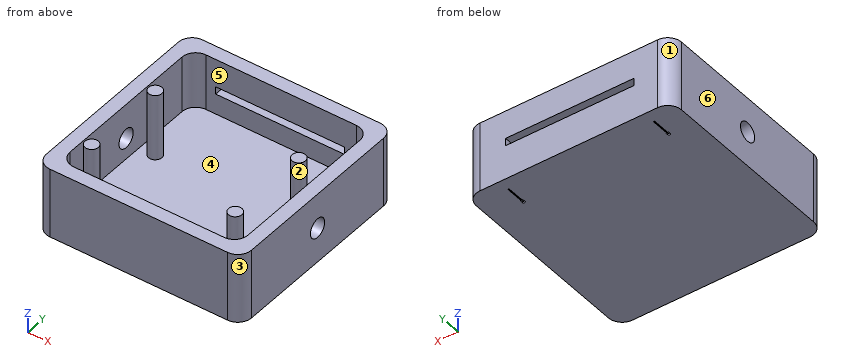
```python
from build123d import *

# Parameters (mm, degrees)
SKETCH1_W           = 30
SKETCH1_H           = 30
BOSS_EXTRUDE1_DEPTH = 2
SKETCH4_R           = 0.9775
BOSS_EXTRUDE3_DEPTH = 9.7
SKETCH5_W           = 30
SKETCH5_H           = 30
SKETCH5_W_2         = 26
SKETCH5_H_2         = 26
BOSS_EXTRUDE4_DEPTH = 8.25
SKETCH6_W           = 18.8
SKETCH6_H           = 1.1
CUT_EXTRUDE1_DEPTH  = 10
FILLET1_R           = 2
CUT_EXTRUDE4_DEPTH  = 0.25
BOSS_EXTRUDE6_DEPTH = 0.05
CUT_EXTRUDE5_DEPTH  = 0.25
BOSS_EXTRUDE7_DEPTH = 0.05
SKETCH23_R          = 1.4
CUT_EXTRUDE6_DEPTH  = 3
CUT_EXTRUDE7_START  = -3
SKETCH24_R          = 1.4
CUT_EXTRUDE7_DEPTH  = 3


with BuildPart() as part:
    # Sketch1 → Boss-Extrude1 (new body)
    with BuildSketch(Plane.XY):
        with Locations((-5.423452769, 0.244299674)):
            Rectangle(SKETCH1_W, SKETCH1_H)
    extrude(amount=BOSS_EXTRUDE1_DEPTH)

    # Sketch4 → Boss-Extrude3 (add)
    with BuildSketch(Plane.XY.offset(2)):
        with Locations((-16.173452769, 2.943299674)):
            Circle(SKETCH4_R)
        with Locations((-16.173452769, -9.555700326)):
            Circle(SKETCH4_R)
        with Locations((4.826547231, 2.943299674)):
            Circle(SKETCH4_R)
        with Locations((4.826547231, -9.555700326)):
            Circle(SKETCH4_R)
    extrude(amount=BOSS_EXTRUDE3_DEPTH)

    # Sketch5 → Boss-Extrude4 (add)
    with BuildSketch(Plane.XY.offset(2)):
        with Locations((-5.423452769, 0.244299674)):
            Rectangle(SKETCH5_W, SKETCH5_H)
        with Locations((-5.423452769, 0.244299674)):
            Rectangle(SKETCH5_W_2, SKETCH5_H_2, mode=Mode.SUBTRACT)
    extrude(amount=BOSS_EXTRUDE4_DEPTH)

    # Sketch6 → Cut-Extrude1 (cut)
    with BuildSketch(Plane(origin=(0, 15.244299674, 0), x_dir=(1, 0, 0), z_dir=(0, 1, 0))):
        with Locations((-5.582175382, -5.564963199)):
            Rectangle(SKETCH6_W, SKETCH6_H)
    extrude(amount=-CUT_EXTRUDE1_DEPTH, mode=Mode.SUBTRACT)

    # Fillet1
    fillet1_edges = [part.edges().sort_by_distance(p)[0] for p in [
        (7.576547231, 13.244299674, 6.125),
        (7.576547231, -12.755700326, 6.125),
        (-18.423452769, -12.755700326, 6.125),
        (-18.423452769, 13.244299674, 6.125),
        (-20.423452769, 15.244299674, 5.125),
        (9.576547231, 15.244299674, 5.125),
        (9.576547231, -14.755700326, 5.125),
        (-20.423452769, -14.755700326, 5.125),
    ]]
    fillet(fillet1_edges, radius=FILLET1_R)

    # Sketch15 → Cut-Extrude4 (cut)
    with BuildSketch(Plane(origin=(0, 0, 0), x_dir=(-1, 0, 0), z_dir=(0, 0, -1))):
        with BuildLine():
            Line((-4.48872314, 13.480732705), (-4.48872314, 10.524770746))
            ThreePointArc((-4.48872314, 10.524770746), (-4.67872314, 10.334770746), (-4.86872314, 10.524770746))
            Line((-4.86872314, 10.524770746), (-4.86872314, 13.480732705))
            ThreePointArc((-4.86872314, 13.480732705), (-4.67872314, 13.670732705), (-4.48872314, 13.480732705))
        make_face()
    extrude(amount=-CUT_EXTRUDE4_DEPTH, mode=Mode.SUBTRACT)

    # Sketch16 → Boss-Extrude6 (add)
    with BuildSketch(Plane(origin=(0, 0, 0), x_dir=(-1, 0, 0), z_dir=(0, 0, -1))):
        with BuildLine():
            Line((-4.86872314, 10.923343064), (-4.772315146, 10.923343064))
            Line((-4.772315146, 10.923343064), (-4.772315146, 13.480732705))
            ThreePointArc((-4.772315146, 13.480732705), (-4.68554888, 13.567498971), (-4.598782614, 13.480732705))
            Line((-4.598782614, 13.480732705), (-4.598782614, 10.923343064))
            Line((-4.598782614, 10.923343064), (-4.48872314, 10.923343064))
            Line((-4.48872314, 10.923343064), (-4.48872314, 13.480732705))
            ThreePointArc((-4.48872314, 13.480732705), (-4.67872314, 13.670732705), (-4.86872314, 13.480732705))
            Line((-4.86872314, 13.480732705), (-4.86872314, 10.923343064))
        make_face()
    extrude(amount=-BOSS_EXTRUDE6_DEPTH)

    # Sketch20 → Cut-Extrude5 (cut)
    with BuildSketch(Plane(origin=(0, 0, 0), x_dir=(-1, 0, 0), z_dir=(0, 0, -1))):
        with BuildLine():
            Line((16.739959819, 13.377498971), (16.739959819, 10.515388846))
            ThreePointArc((16.739959819, 10.515388846), (16.549959819, 10.325388846), (16.359959819, 10.515388846))
            Line((16.359959819, 10.515388846), (16.359959819, 13.377498971))
            ThreePointArc((16.359959819, 13.377498971), (16.549959819, 13.567498971), (16.739959819, 13.377498971))
        make_face()
    extrude(amount=-CUT_EXTRUDE5_DEPTH, mode=Mode.SUBTRACT)

    # Sketch19 → Boss-Extrude7 (add)
    with BuildSketch(Plane(origin=(0, 0, 0), x_dir=(-1, 0, 0), z_dir=(0, 0, -1))):
        with BuildLine():
            Line((16.359959819, 10.82010933), (16.456367814, 10.82010933))
            Line((16.456367814, 10.82010933), (16.456367814, 13.377498971))
            ThreePointArc((16.456367814, 13.377498971), (16.543134079, 13.464265237), (16.629900345, 13.377498971))
            Line((16.629900345, 13.377498971), (16.629900345, 10.82010933))
            Line((16.629900345, 10.82010933), (16.739959819, 10.82010933))
            Line((16.739959819, 10.82010933), (16.739959819, 13.377498971))
            ThreePointArc((16.739959819, 13.377498971), (16.549959819, 13.567498971), (16.359959819, 13.377498971))
            Line((16.359959819, 13.377498971), (16.359959819, 10.82010933))
        make_face()
    extrude(amount=-BOSS_EXTRUDE7_DEPTH)

    # Sketch23 → Cut-Extrude6 (cut)
    with BuildSketch(Plane.ZY.offset(20.423452769)):
        with Locations((5.125, 0.244299674)):
            Circle(SKETCH23_R)
    extrude(amount=-CUT_EXTRUDE6_DEPTH, mode=Mode.SUBTRACT)

    # Sketch24 → Cut-Extrude7 (cut)
    with BuildSketch(Plane(origin=(9.576547231, 0, 0), x_dir=(0, 0, -1), z_dir=(1, 0, 0)).offset(CUT_EXTRUDE7_START)):
        with Locations(Location((-5.125, 0.244299674, 0), (0, 0, 180))):
            Circle(SKETCH24_R)
    extrude(amount=CUT_EXTRUDE7_DEPTH, mode=Mode.SUBTRACT)


solid = part.part
```
Input: part model. Units: mm. Frame: model coordinates. Face numbers are marked on the shaded views. A direction names the side the tool comes from. Coordinates: 2 decimals unless noted, no trailing zeros. Loops run counter-clockwise (first coordinate to the right, second up) from the corner with the lowest first, then second, coordinate; pieces in that order, holes last. Notation, with made-up numbers: (54.25, 5.5) - (108.25, 5.5) arc R17 ccw to (108.25, 23.5) - close; hole circle Ø9 at (3, -6). An arc over 180 degrees is marked (long way). Answer in a Markdown table with one row per item.
(1) Cut plane A-A on x = -11.75. Output: boundary loops of the cut face in (y, z).
Model answer:
| item | result |
|---|---|
| outline | (-14.76, 0) - (15.24, 0) - (15.24, 5.01) - (13.24, 5.01) - (13.24, 2) - (-12.76, 2) - (-12.76, 10.25) - (-14.76, 10.25) - close; (13.24, 6.11) - (15.24, 6.11) - (15.24, 10.25) - (13.24, 10.25) - close |
(2) Mould query, pull axis X, two halves, no side actions, for the marked faces 1, 2, 3 and 4. Classes: pulls with the +X half, pulls with the -X half, needs draft (parallel to the pull), parting line crosses it, or undercut.
Model answer:
| item | result |
|---|---|
| face 1 | pulls with the -X half |
| face 2 | undercut |
| face 3 | pulls with the +X half |
| face 4 | undercut |
(3) Cut plane C-C on y = -4. Output: boundary loops of the cut face in (x, z).
Model answer:
| item | result |
|---|---|
| outline | (-20.42, 0) - (9.58, 0) - (9.58, 10.25) - (7.58, 10.25) - (7.58, 2) - (-18.42, 2) - (-18.42, 10.25) - (-20.42, 10.25) - close |
(4) Pin query (flat end, axial travel): P1, Ø8, axis at x = -6, y = -3.5, coming from the +Z side; P2, Ø2, axis at y = 0.24, z = 5.12, coming from the -X side; P3, Ø6, axis at x = -4, y = -11, coming from the +Z side; P4, Ø0.5, axis at y = 14.5, z = 5.5, coming from the +X side. Return the tip coordinate at first contact, or that it passes through.
Model answer:
| item | result |
|---|---|
| P1 | stops at z = 2 |
| P2 | passes through |
| P3 | stops at z = 10.25 |
| P4 | stops at x = 9.31 |
(5) Cut plane D-D on z = 4.25. Output: boundary loops of the cut face in (x, y) (1 decimal).
Model answer:
| item | result |
|---|---|
| outline | (-20.4, -12.8) arc R2 ccw to (-18.4, -14.8) - (7.6, -14.8) arc R2 ccw to (9.6, -12.8) - (9.6, -0.8) - (7.6, -0.8) - (7.6, -10.8) arc R2 cw to (5.6, -12.8) - (-16.4, -12.8) arc R2 cw to (-18.4, -10.8) - (-18.4, -0.8) - (-20.4, -0.8) - close; (-20.4, 1.3) - (-18.4, 1.3) - (-18.4, 11.2) arc R2 cw to (-16.4, 13.2) - (5.6, 13.2) arc R2 cw to (7.6, 11.2) - (7.6, 1.3) - (9.6, 1.3) - (9.6, 13.2) arc R2 ccw to (7.6, 15.2) - (-18.4, 15.2) arc R2 ccw to (-20.4, 13.2) - close; circle Ø2 at (-16.2, -9.6); circle Ø2 at (-16.2, 2.9); circle Ø2 at (4.8, -9.6); circle Ø2 at (4.8, 2.9) |
(6) Material intervals for L1, parallel to X at y = -2.5, z = 5.75; L2, parallel to Y at x = 0, z = 10; L3, parallel to Y at x = -15.5, z = 8.5, sorted ascending. Write a range as from..to.
Model answer:
| item | result |
|---|---|
| L1 | x = -20.42..-18.42, 7.58..9.58 |
| L2 | y = -14.76..-12.76, 13.24..15.24 |
| L3 | y = -14.76..-12.76, -10.26..-8.85, 2.23..3.65, 13.24..15.24 |
(7) Cut plane B-B on z = 9. Output: boundary loops of the cut face in (x, y) (1 decimal).
Model answer:
| item | result |
|---|---|
| outline | (-20.4, -12.8) arc R2 ccw to (-18.4, -14.8) - (7.6, -14.8) arc R2 ccw to (9.6, -12.8) - (9.6, 13.2) arc R2 ccw to (7.6, 15.2) - (-18.4, 15.2) arc R2 ccw to (-20.4, 13.2) - close; circle Ø2 at (-16.2, -9.6); circle Ø2 at (-16.2, 2.9); circle Ø2 at (4.8, -9.6); circle Ø2 at (4.8, 2.9); hole (-18.4, -10.8) arc R2 ccw to (-16.4, -12.8) - (5.6, -12.8) arc R2 ccw to (7.6, -10.8) - (7.6, 11.2) arc R2 ccw to (5.6, 13.2) - (-16.4, 13.2) arc R2 ccw to (-18.4, 11.2) - close |
(8) Set-up query: the marked faces 5 and 6. Return all of +Z, -Z, +X, -X, +Y, -Y with unobstructed straight access to the full face (end or side cutting, diameter ignored); none if empty.
Model answer:
| item | result |
|---|---|
| face 5 | +Z |
| face 6 | +Z, -Z, -X, +Y, -Y |
